Could you check a few things on this model? Use its own coordinates, in mm. A direction names the side the tool comes from. Coordinates: 2 decimals unless noted, no trailing zeros. Order: outer loops, then holes, each group sorted by start corner. A loop starts at its lowest first (then second) coordinate and runs counter-clockwise, first axis right, second up. Notation, with made-up numbers: (88, -7.75) -> (119, -7.75) arc R30 cw to (119, 18.25) -> close; hole circle Ø8 at (0, 37.25). An arc over 180 degrees is marked (long way). Use a Markdown table: item, result. Add a question column.
1) Will these pins go through, and if not, where does the flat tip stop? pin 1 Ø3 at (x, z) = (-4.5, 2) entering from -Y; pin 2 Ø3 at (x, y) = (-5.5, -2.5) entering from -Z; pin 3 Ø1.2 at (x, z) = (-38, 2.5) entering from +Y.
2) Thinking about a two-plate mould opening in Y: for faces 1 (the flat face through (-39.6, -35.7, 4)), 2 (the flat face through (-40, -6.016, 2)), 3 (the cylindrical face through (-31.757, -21.237, 3.451)), which applies, +Y half, -Y half, draft (parallel to the pull), parting line (faces both ways), or undercut?
3) Which directions (+Z, -Z, +X, -X, +Y, -Y) give clear straight access to the entire face, cutting with the end or side of a thin tool? Please do faces 4 (the flat face through (-36.544, -3, 2)), 5 (the flat face through (-8.544, -37, 2)), 6 (the flat face through (-40, -34.016, 2)), 7 (the cylindrical face through (-41.67, -37.45, 5.48)), 8 (the flat face through (-8.544, -3, 2)).
4) If we section it at A-A (x = -40): Write out the boundary of the cut face in (y, z).
5) If we section it at B-B (y = -35): Write out the boundary of the cut face in (x, z).
6) If we section it at D-D (z = 3): Write out the boundary of the cut face in (x, y).
7) If I drill on L1, parallel to Y at x = -5, z = 6.5; L2, parallel to Y at x = -39.5, z = 5.5; L3, parallel to X at y = -19, z = 5.5, over which ranges is the centre line in solid material (lowest first)? Write a range as [from, to].
8) If we section it at C-C (z = 6): Write out the boundary of the cut face in (x, y).
```python
from build123d import *

# Parameters (mm, degrees)
F0_W     = 40
F0_H     = 40
F0_R     = 1.6256
F0_R_2   = 2.0066
F1_DEPTH = 7
F2_W     = 6
F2_H     = 6
F2_R     = 1.6256
F3_DEPTH = 4


with BuildPart() as f1:
    # F0 (on Top) → F1 (new body)
    with BuildSketch(Plane.XY):
        with Locations((-22.544218, -20.016475)):
            Rectangle(F0_W, F0_H)
        with Locations((-40.044218, -37.516475)):
            Circle(F0_R, mode=Mode.SUBTRACT)
        with Locations((-5.044218, -37.516475)):
            Circle(F0_R, mode=Mode.SUBTRACT)
        with Locations((-30.164218, -20.016475)):
            Circle(F0_R_2, mode=Mode.SUBTRACT)
        with Locations((-40.044218, -2.516475)):
            Circle(F0_R, mode=Mode.SUBTRACT)
        with Locations((-14.924218, -20.016475)):
            Circle(F0_R_2, mode=Mode.SUBTRACT)
        with Locations((-5.044218, -2.516475)):
            Circle(F0_R, mode=Mode.SUBTRACT)
    extrude(amount=F1_DEPTH)

    # F2 (on face) → F3 (cut)
    with BuildSketch(Plane(origin=(0, 0, 0), x_dir=(1, 0, 0), z_dir=(0, 0, -1))):
        with Locations((-39.544218, 37.016475)):
            Rectangle(F2_W, F2_H)
        with Locations((-40.044218, 37.516475)):
            Circle(F2_R, mode=Mode.SUBTRACT)
        with Locations((-5.544218, 37.016475)):
            Rectangle(F2_W, F2_H)
        with Locations((-5.044218, 37.516475)):
            Circle(F2_R, mode=Mode.SUBTRACT)
        with Locations((-5.544218, 3.016475)):
            Rectangle(F2_W, F2_H)
        with Locations((-5.044218, 2.516475)):
            Circle(F2_R, mode=Mode.SUBTRACT)
        with Locations((-39.544218, 3.016475)):
            Rectangle(F2_W, F2_H)
        with Locations((-40.044218, 2.516475)):
            Circle(F2_R, mode=Mode.SUBTRACT)
    extrude(amount=-F3_DEPTH, mode=Mode.SUBTRACT)


solid = f1.part
```
Answer sheet:
| question | item | result |
|---|---|---|
| 1 | pin 1 | y = -34.02 |
| 1 | pin 2 | z = 4 |
| 1 | pin 3 | y = -6.02 |
| 2 | face 1 | draft |
| 2 | face 2 | +Y half |
| 2 | face 3 | undercut |
| 3 | face 4 | -Z, -X, +Y |
| 3 | face 5 | -Z, +X, -Y |
| 3 | face 6 | -Z, -X, -Y |
| 3 | face 7 | +Z, -Z |
| 3 | face 8 | -Z, +X, +Y |
| 4 | outline | (-40.02, 4) -> (-39.14, 4) -> (-39.14, 7) -> (-40.02, 7) -> close; (-35.89, 4) -> (-34.02, 4) -> (-34.02, 0) -> (-6.02, 0) -> (-6.02, 4) -> (-4.14, 4) -> (-4.14, 7) -> (-35.89, 7) -> close; (-0.89, 4) -> (-0.02, 4) -> (-0.02, 7) -> (-0.89, 7) -> close |
| 5 | outline | (-42.54, 4) -> (-36.54, 4) -> (-36.54, 0) -> (-8.54, 0) -> (-8.54, 4) -> (-2.54, 4) -> (-2.54, 7) -> (-42.54, 7) -> close |
| 6 | outline | (-42.54, -34.02) -> (-36.54, -34.02) -> (-36.54, -40.02) -> (-8.54, -40.02) -> (-8.54, -34.02) -> (-2.54, -34.02) -> (-2.54, -6.02) -> (-8.54, -6.02) -> (-8.54, -0.02) -> (-36.54, -0.02) -> (-36.54, -6.02) -> (-42.54, -6.02) -> close; hole circle Ø4.01 at (-30.16, -20.02); hole circle Ø4.01 at (-14.92, -20.02) |
| 7 | L1 | [-40.02, -39.14], [-35.89, -4.14], [-0.89, -0.02] |
| 7 | L2 | [-40.02, -39.05], [-35.98, -4.05], [-0.98, -0.02] |
| 7 | L3 | [-42.54, -31.89], [-28.43, -16.65], [-13.19, -2.54] |
| 8 | outline | (-42.54, -40.02) -> (-2.54, -40.02) -> (-2.54, -0.02) -> (-42.54, -0.02) -> close; hole circle Ø3.25 at (-40.04, -37.52); hole circle Ø3.25 at (-40.04, -2.52); hole circle Ø4.01 at (-30.16, -20.02); hole circle Ø4.01 at (-14.92, -20.02); hole circle Ø3.25 at (-5.04, -37.52); hole circle Ø3.25 at (-5.04, -2.52) |
